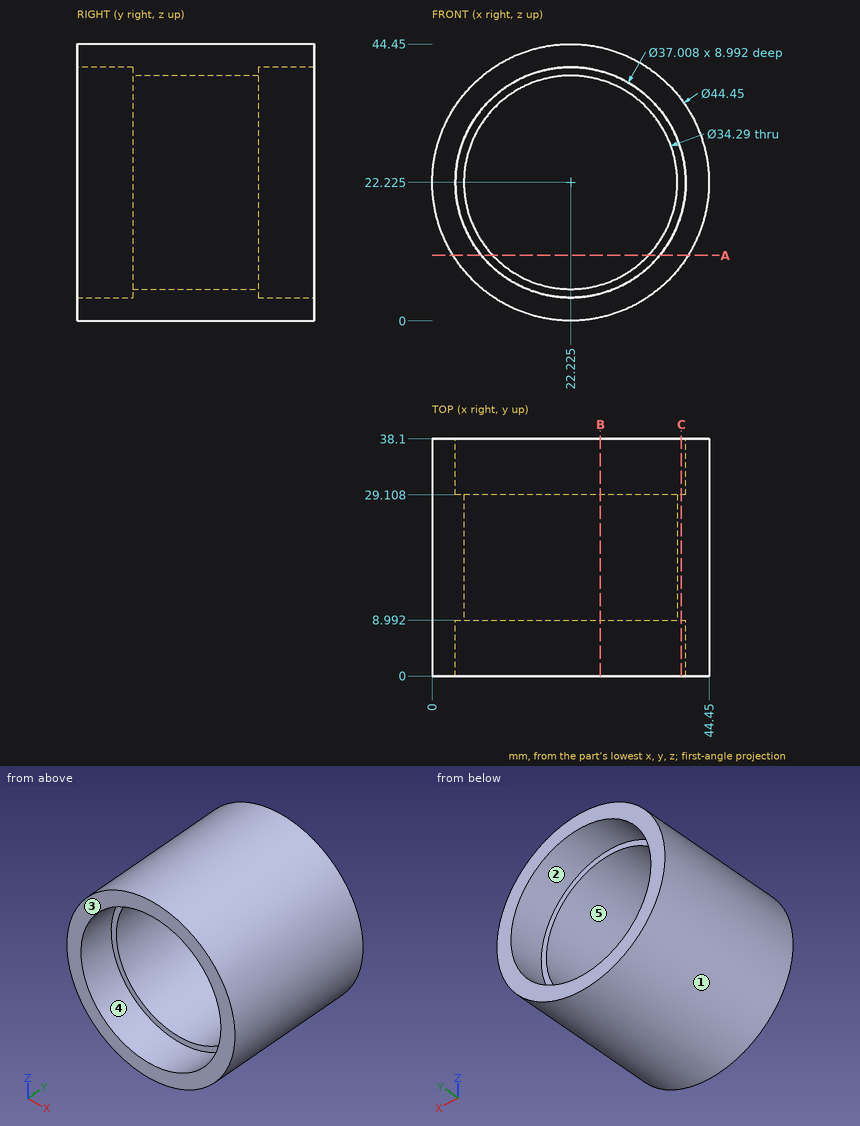
Job drawing, mm, ordinate dimensions from the low corner. One solid piece. A direction names the side the tool comes from. Give positions to 0.01 mm unless a question says otherwise; leave off trailing zeros. Write each loop counter-clockwise with the first axis right and the second up, starting at its lowest first coordinate (ties: lowest second). Pieces come first, ordered by that corner, then holes. Notation, with made-up numbers: (42, -24.5) - (87, -24.5) arc R22 ccw to (87, 14.5) - close; hole circle Ø7 at (26.5, 57.5). An arc over 180 degrees is marked (long way). Use one line per item in the form item = value. Start each with the question number.
1. Two-plate mould, pull along Z, no slides. Class the marked faces 1, 2 and 3: released by +Z, released by -Z, zero draft, split by the parting line, or undercut.
2. 3-axis set-ups, long thin cutter, end or side, ignore diameter. For the marked faces 4 and 5: which of +Z, -Z, +X, -X, +Y, -Y reach the whole face in a straight line?
3. Band-saw the part on A-A on z = 10.5. Write the cut outline in (x, y) (1 decimal).
4. Drop flat-ended pins along their axis: pin 1 Ø5 at (x, y) = (11.5, 15) entering from +Z; pin 2 Ø18.5 at (x, z) = (14.5, 19.5) entering from -Y; pin 3 Ø8 at (y, z) = (24.5, 19.5) entering from -X. Give the stop position or say it passes through.
5. Band-saw the part on B-B on x = 27. Write the cut outline in (y, z).
6. Band-saw the part on C-C on x = 40. Write the cut outline in (y, z).
7. Probe line 1 (Z direction, x = 22.5, y = 23); line 2 (Z direction, x = 20.5, y = 4); line 3 (X direction, y = 10, z = 30.5). List the from-to ranges inside material, lowest first. Write a range as [from, to].
Conclusion:
q1.face_1 = split by the parting line
q1.face_2 = undercut
q1.face_3 = zero draft
q2.face_4 = -Y
q2.face_5 = +Y, -Y
q3.outline = (3.3, 0) - (7.9, 0) - (7.9, 9) - (9.7, 9) - (9.7, 29.1) - (7.9, 29.1) - (7.9, 38.1) - (3.3, 38.1) - close; (34.7, 9) - (36.5, 9) - (36.5, 0) - (41.1, 0) - (41.1, 38.1) - (36.5, 38.1) - (36.5, 29.1) - (34.7, 29.1) - close
q4.pin_1 = 42.87
q4.pin_2 = 8.99
q4.pin_3 = 0
q5.outline = (0, 0.52) - (38.1, 0.52) - (38.1, 4.35) - (29.11, 4.35) - (29.11, 5.76) - (8.99, 5.76) - (8.99, 4.35) - (0, 4.35) - close; (0, 40.1) - (8.99, 40.1) - (8.99, 38.69) - (29.11, 38.69) - (29.11, 40.1) - (38.1, 40.1) - (38.1, 43.93) - (0, 43.93) - close
q6.outline = (0, 8.88) - (38.1, 8.88) - (38.1, 17.08) - (29.11, 17.08) - (29.11, 27.37) - (38.1, 27.37) - (38.1, 35.57) - (0, 35.57) - (0, 27.37) - (8.99, 27.37) - (8.99, 17.08) - (0, 17.08) - close
q7.line_1 = [0, 5.08], [39.37, 44.45]
q7.line_2 = [0.07, 3.8], [40.65, 44.38]
q7.line_3 = [1.6, 7.21], [37.24, 42.85]
